For this review, use the dimensioned drawing (mm, ordinates from the lowest corner) and the shaded views. Give positions to 0.01 mm unless a question says otherwise; leave off trailing zeros. Write each loop counter-clockwise with the first axis right and the second up, starting at its lowest first coordinate (ties: lowest second). Pieces come first, ordered by that corner, then holes. Notation, with made-up numbers: (6, -13.5) - (15, -13.5) arc R16 cw to (15, 11.5) - close; hole circle Ø3 at (72, 62.25). An arc over 180 degrees is marked (long way). Use a Markdown table: item, result. Add a question column.
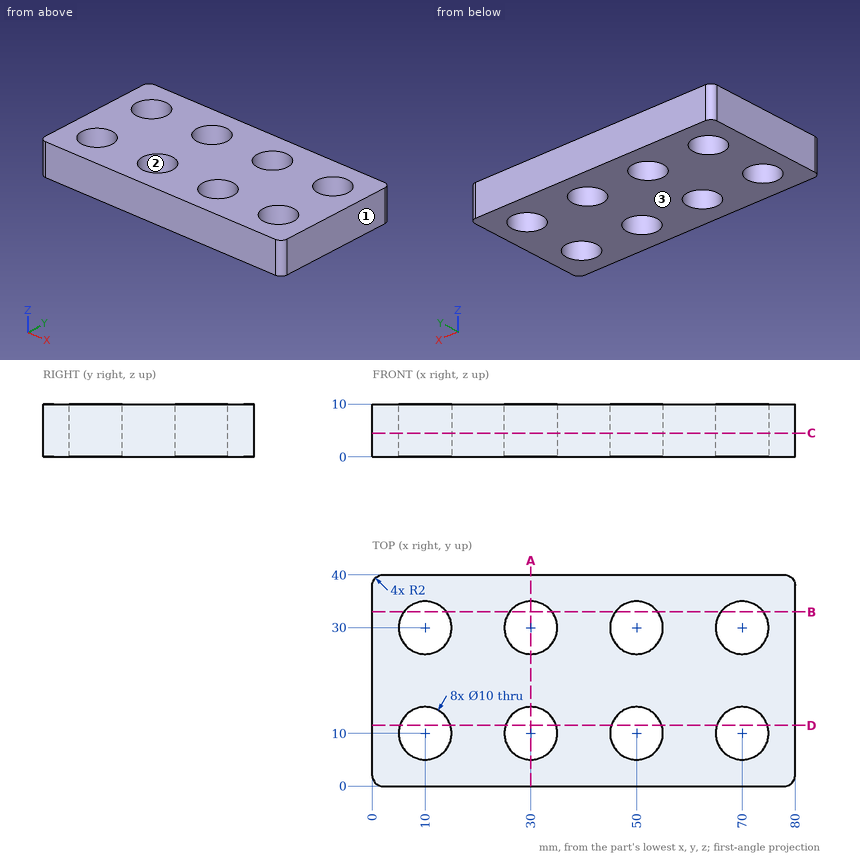
(1) Add section C-C (z = 4.5). Count the separate pieces of the cut face and the enclosed holes in it, and give its area (3 significant figures).
(2) Mouldability with a two-part tool opening along X and no side actions: class the marked faces 1, 2 and 3 as +X half, -X half, draft (parallel to the pull), parting line (faces both ways), or undercut.
(3) Add section A-A (x = 30). State the section outline as (y, z) points, and give its area (3 significant figures).
(4) Add section B-B (y = 33). State the section outline as (x, z) points.
(5) Insertion check: pin 1 (8 mm diameter, centred on x = 10, y = 30, fed in from +Z). The pin has a flat end and moves straight along its axis. Give the tip position at first contact, or say it passes through.
(6) Add section D-D (y = 11.5). State the section outline as (x, z) points, and give its area (3 significant figures).
(7) For line 1 along Y through (x, z) = (30, 9.5); line 2 along Y through (x, z) = (53.5, 1); line 3 along X through (y, z) = (34, 8), list the stretches that pass through material, from the lowest coordinate up.
Answers follow:
| question | item | result |
|---|---|---|
| 1 | separate pieces | 1 |
| 1 | enclosed holes | 8 |
| 1 | area | 2,570 mm^2 |
| 2 | face 1 | +X half |
| 2 | face 2 | undercut |
| 2 | face 3 | draft |
| 3 | outline | (0, 0) - (5, 0) - (5, 10) - (0, 10) - close; (15, 0) - (25, 0) - (25, 10) - (15, 10) - close; (35, 0) - (40, 0) - (40, 10) - (35, 10) - close |
| 3 | area | 200 mm^2 |
| 4 | outline | (0, 0) - (6, 0) - (6, 10) - (0, 10) - close; (14, 0) - (26, 0) - (26, 10) - (14, 10) - close; (34, 0) - (46, 0) - (46, 10) - (34, 10) - close; (54, 0) - (66, 0) - (66, 10) - (54, 10) - close; (74, 0) - (80, 0) - (80, 10) - (74, 10) - close |
| 5 | pin 1 | through |
| 6 | outline | (0, 0) - (5.23, 0) - (5.23, 10) - (0, 10) - close; (14.77, 0) - (25.23, 0) - (25.23, 10) - (14.77, 10) - close; (34.77, 0) - (45.23, 0) - (45.23, 10) - (34.77, 10) - close; (54.77, 0) - (65.23, 0) - (65.23, 10) - (54.77, 10) - close; (74.77, 0) - (80, 0) - (80, 10) - (74.77, 10) - close |
| 6 | area | 418 mm^2 |
| 7 | line 1 | 0 to 5, 15 to 25, 35 to 40 |
| 7 | line 2 | 0 to 6.43, 13.57 to 26.43, 33.57 to 40 |
| 7 | line 3 | 0 to 7, 13 to 27, 33 to 47, 53 to 67, 73 to 80 |
